Read the model definition and answer for the solid it produces. Units are mm, in the model's axes. A direction names the side the tool comes from. Give positions to 0.01 mm unless a question says otherwise; leave off trailing zeros. Loops run counter-clockwise (first coordinate to the right, second up) from the corner with the lowest first, then second, coordinate; pieces in that order, holes last. Notation, with made-up numbers: (14, -33.5) - (18, -33.5) arc R22 ccw to (18, -4.5) - close; hole circle Ø5 at (15, 44.5). An arc over 180 degrees is marked (long way). Write each question's results on one line, items separated by ' | '. Start each with the question number.
Q1. Determine the mould class of faces 4 (the cylindrical face through (39.563, 38.418, -54.93)), 5 (the flat face through (35.7, 37.6, -30)), 6 (the flat face through (37, 30, -40)), 7 (the flat face through (37, 35, -25)) for opening direction Z: +Z half, -Z half, draft (parallel to the pull), parting line (faces both ways), or undercut.
Q2. The part is cut by section B-B, the plane x = 37.5. Write down the section's boundary in (y, z).
Q3. Find the intervals of material crossed by line 1 (Z direction, x = 37.5, y = 45); line 2 (Y direction, x = 37.5, z = -52.25); line 3 (Y direction, x = 11, z = -52), in increasing order. Write a range as from..to.
Q4. The part is cut by section C-C, the plane y = 40. Write down the section's boundary in (x, z).
Q5. The part is cut by section A-A, the plane z = -37.5. Write down the section's boundary in (x, y).
Q6. For faces 1 (the cylindrical face through (31.5, 24.4, -37.3)), 2 (the flat face through (30, 13, -38)), 3 (the flat face through (17, 5, -80)), determine the directions among +Z, -Z, +X, -X, +Y, -Y from which every point of the face is accessible in a straight line to the end or side of a thin tool.
Q7. The part is cut by section D-D, the plane y = 7. Write down the section's boundary in (x, z), plus the area to 3 significant figures.
Q8. Given pin 1 (10 mm diameter, centred on x = 37.5, y = 26.5, fed in from +Z); pin 2 (1.8 mm diameter, centred on y = 60.5, z = -35.5, fed in from -X); pin 3 (7.5 mm diameter, centred on x = 37.5, y = 39, fed in from -Z), each flat-ended and moving along its own axis, determine where each tip first touches the part or whether it passes through.
```python
from build123d import *

# Parameters (mm, degrees)
SKETCH4_W               = 40
SKETCH4_H               = 80
BOSS_EXTRUDE4_DEPTH     = 5
SKETCH5_W               = 10
SKETCH5_H               = 5
BOSS_EXTRUDE6_DEPTH     = 50
SKETCH7_W               = 10
SKETCH7_H               = 25
SKETCH7_H_2             = 5
BOSS_EXTRUDE7_DEPTH     = 20
SKETCH8_W               = 40
SKETCH8_H               = 5
BOSS_EXTRUDE8_DEPTH     = 20
SKETCH9_W               = 100
SKETCH9_H               = 5
BOSS_EXTRUDE9_DEPTH     = 10
SKETCH10_W              = 5
SKETCH10_H              = 50
BOSS_EXTRUDE10_DEPTH    = 40
BOSS_EXTRUDE11_DEPTH    = 10
SKETCH12_R              = 15
SKETCH12_R_2            = 1.8
CUT_EXTRUDE1_DEPTH      = 5
CUT_EXTRUDE2_DEPTH      = 92.241437954
CUT_EXTRUDE2_DEPTH_BACK = 92.241437954
SKETCH13_R              = 2.25
SKETCH14_R              = 4
SKETCH14_R_2            = 2.25
CUT_EXTRUDE4_DEPTH      = 2
CUT_EXTRUDE5_START      = -2
SKETCH15_R              = 4
SKETCH15_R_2            = 2.25
CUT_EXTRUDE5_DEPTH      = 2
SKETCH17_R              = 5
CUT_EXTRUDE6_DEPTH      = 25
SKETCH19_W              = 50
SKETCH19_H              = 60
SKETCH19_R              = 1.8
SKETCH19_R_2            = 15
SKETCH19_R_3            = 4
BOSS_EXTRUDE13_DEPTH    = 5
SKETCH20_R              = 4
SKETCH20_R_2            = 2.25
BOSS_EXTRUDE14_DEPTH    = 5
SKETCH21_W              = 20
SKETCH21_H              = 20
BOSS_EXTRUDE15_DEPTH    = 5
BOSS_EXTRUDE16_START    = -10
SKETCH22_R              = 4
BOSS_EXTRUDE16_DEPTH    = 10
SKETCH23_R              = 4
BOSS_EXTRUDE17_DEPTH    = 5
CUT_EXTRUDE7_DEPTH      = 106.59356041
CUT_EXTRUDE7_DEPTH_BACK = 106.59356041
SKETCH24_R              = 2.6


with BuildPart() as part:
    # Sketch4 → Boss-Extrude4 (new body)
    with BuildSketch(Plane(origin=(0, 0, 0), x_dir=(1, 0, 0), z_dir=(0, 1, 0))):
        with Locations((20, 40)):
            Rectangle(SKETCH4_W, SKETCH4_H)
    extrude(amount=BOSS_EXTRUDE4_DEPTH)

    # Sketch5 → Boss-Extrude6 (add)
    with BuildSketch(Plane(origin=(0, 5, 0), x_dir=(1, 0, 0), z_dir=(0, 1, 0))):
        with Locations((35, 52.5)):
            Rectangle(SKETCH5_W, SKETCH5_H)
        with Locations((35, 27.5)):
            Rectangle(SKETCH5_W, SKETCH5_H)
    extrude(amount=BOSS_EXTRUDE6_DEPTH)

    # Sketch7 → Boss-Extrude7 (add)
    with BuildSketch(Plane.XY.offset(-50)):
        with Locations((35, 17.5)):
            Rectangle(SKETCH7_W, SKETCH7_H)
        with Locations((35, 52.5)):
            Rectangle(SKETCH7_W, SKETCH7_H_2)
    extrude(amount=BOSS_EXTRUDE7_DEPTH)

    # Sketch8 → Boss-Extrude8 (add)
    with BuildSketch(Plane(origin=(0, 0, -80), x_dir=(-1, 0, 0), z_dir=(0, 0, -1))):
        with Locations((-20, 2.5)):
            Rectangle(SKETCH8_W, SKETCH8_H)
    extrude(amount=BOSS_EXTRUDE8_DEPTH)

    # Sketch9 → Boss-Extrude9 (add)
    with BuildSketch(Plane.ZY):
        with Locations((-50, 2.5)):
            Rectangle(SKETCH9_W, SKETCH9_H)
    extrude(amount=BOSS_EXTRUDE9_DEPTH)

    # Sketch10 → Boss-Extrude10 (add)
    with BuildSketch(Plane.ZY.offset(-30)):
        with Locations((-52.5, 30)):
            Rectangle(SKETCH10_W, SKETCH10_H)
    extrude(amount=BOSS_EXTRUDE10_DEPTH)

    # Sketch11 → Boss-Extrude11 (add)
    with BuildSketch(Plane(origin=(0, 55, 0), x_dir=(1, 0, 0), z_dir=(0, 1, 0))):
        Polygon((40, 55), (-10, 55), (-10, 50), (30, 50), (30, 25), (40, 25), align=None)
    extrude(amount=BOSS_EXTRUDE11_DEPTH)

    # Sketch12 → Cut-Extrude1 (cut)
    with BuildSketch(Plane.XY.offset(-50)):
        with Locations((11, 40)):
            Circle(SKETCH12_R)
        with Locations((-4.499780644, 55.499780644)):
            Circle(SKETCH12_R_2)
        with Locations((26.499780644, 55.499780644)):
            Circle(SKETCH12_R_2)
        with Locations((-4.499780644, 24.500219356)):
            Circle(SKETCH12_R_2)
        with Locations((26.499780644, 24.500219356)):
            Circle(SKETCH12_R_2)
    extrude(amount=-CUT_EXTRUDE1_DEPTH, mode=Mode.SUBTRACT)

    # Sketch13 → Cut-Extrude2 (cut, two sides: drawn at the far end of the back side and taken through both)
    with BuildSketch(Plane.XY.offset(-50).offset(-CUT_EXTRUDE2_DEPTH_BACK)):
        with Locations((35, 40)):
            Circle(SKETCH13_R)
    extrude(amount=CUT_EXTRUDE2_DEPTH + CUT_EXTRUDE2_DEPTH_BACK, mode=Mode.SUBTRACT)

    # Sketch14 → Cut-Extrude4 (cut)
    with BuildSketch(Plane.XY.offset(-25)):
        with Locations((35, 40)):
            Circle(SKETCH14_R)
        with Locations((35, 40)):
            Circle(SKETCH14_R_2, mode=Mode.SUBTRACT)
    extrude(amount=-CUT_EXTRUDE4_DEPTH, mode=Mode.SUBTRACT)

    # Sketch15 → Cut-Extrude5 (cut)
    with BuildSketch(Plane(origin=(0, 0, -55), x_dir=(-1, 0, 0), z_dir=(0, 0, -1)).offset(CUT_EXTRUDE5_START)):
        with Locations(Location((-35, 40, 0), (0, 0, 180))):
            Circle(SKETCH15_R)
        with Locations(Location((-35, 40, 0), (0, 0, 180))):
            Circle(SKETCH15_R_2, mode=Mode.SUBTRACT)
    extrude(amount=CUT_EXTRUDE5_DEPTH, mode=Mode.SUBTRACT)

    # Sketch17 → Cut-Extrude6 (cut)
    with BuildSketch(Plane.XY.offset(-25)):
        with Locations((26.499780644, 55.499780644)):
            Circle(SKETCH17_R)
        with Locations((26.499780644, 24.500219356)):
            Circle(SKETCH17_R)
    extrude(amount=-CUT_EXTRUDE6_DEPTH, mode=Mode.SUBTRACT)

    # Sketch19 → Boss-Extrude13 (add)
    with BuildSketch(Plane(origin=(0, 0, -55), x_dir=(-1, 0, 0), z_dir=(0, 0, -1))):
        with Locations((-15, 35)):
            Rectangle(SKETCH19_W, SKETCH19_H)
        with Locations(Location((4.499780644, 55.499780644, 0), (0, 0, 180))):
            Circle(SKETCH19_R, mode=Mode.SUBTRACT)
        with Locations(Location((4.499780644, 24.500219356, 0), (0, 0, 180))):
            Circle(SKETCH19_R, mode=Mode.SUBTRACT)
        with Locations(Location((-26.499780644, 24.500219356, 0), (0, 0, 180))):
            Circle(SKETCH19_R, mode=Mode.SUBTRACT)
        with Locations(Location((-11, 40, 0), (0, 0, 180))):
            Circle(SKETCH19_R_2, mode=Mode.SUBTRACT)
        with Locations(Location((-35, 40, 0), (0, 0, 180))):
            Circle(SKETCH19_R_3, mode=Mode.SUBTRACT)
        with Locations(Location((-26.499780644, 55.499780644, 0), (0, 0, 180))):
            Circle(SKETCH19_R, mode=Mode.SUBTRACT)
    extrude(amount=BOSS_EXTRUDE13_DEPTH)

    # Sketch20 → Boss-Extrude14 (add)
    with BuildSketch(Plane(origin=(0, 0, -53), x_dir=(-1, 0, 0), z_dir=(0, 0, -1))):
        with Locations(Location((-35, 40, 0), (0, 0, 180))):
            Circle(SKETCH20_R)
        with Locations(Location((-35, 40, 0), (0, 0, 180))):
            Circle(SKETCH20_R_2, mode=Mode.SUBTRACT)
    extrude(amount=BOSS_EXTRUDE14_DEPTH)

    # Sketch21 → Boss-Extrude15 (add)
    with BuildSketch(Plane(origin=(40, 0, 0), x_dir=(0, 0, -1), z_dir=(1, 0, 0))):
        Polygon((100, 5), (60, 5), (60, 65), (25, 65), (25, 5), (0, 5), (0, 0), (100, 0), align=None)
        with Locations((40, 40)):
            Rectangle(SKETCH21_W, SKETCH21_H, mode=Mode.SUBTRACT)
    extrude(amount=BOSS_EXTRUDE15_DEPTH)

    # Sketch22 → Boss-Extrude16 (add)
    with BuildSketch(Plane(origin=(0, 0, -60), x_dir=(-1, 0, 0), z_dir=(0, 0, -1)).offset(BOSS_EXTRUDE16_START)):
        with Locations(Location((-35, 40, 0), (0, 0, 180))):
            Circle(SKETCH22_R)
    extrude(amount=BOSS_EXTRUDE16_DEPTH)

    # Sketch23 → Boss-Extrude17 (add)
    with BuildSketch(Plane.XY.offset(-25)):
        with Locations((35, 40)):
            Circle(SKETCH23_R)
    extrude(amount=-BOSS_EXTRUDE17_DEPTH)

    # Sketch24 → Cut-Extrude7 (cut, two sides: drawn at the far end of the back side and taken through both)
    with BuildSketch(Plane(origin=(0, 0, -30), x_dir=(-1, 0, 0), z_dir=(0, 0, -1)).offset(-CUT_EXTRUDE7_DEPTH_BACK)):
        with Locations((-37.5, 40)):
            Circle(SKETCH24_R)
    extrude(amount=CUT_EXTRUDE7_DEPTH + CUT_EXTRUDE7_DEPTH_BACK, mode=Mode.SUBTRACT)


solid = part.part
```
Check sheet entries:
1) face 4: draft | face 5: undercut | face 6: undercut | face 7: +Z half
2) outline: (0, -100) - (5, -100) - (5, -60) - (37.4, -60) - (37.4, -50) - (30, -50) - (30, -30) - (37.4, -30) - (37.4, -25) - (5, -25) - (5, 0) - (0, 0) - close; (42.6, -60) - (65, -60) - (65, -25) - (42.6, -25) - (42.6, -30) - (50, -30) - (50, -50) - (42.6, -50) - close
3) line 1: z = -60..-50, -30..-25 | line 2: y = 0..37.4, 42.6..65 | line 3: y = 0..25, 55..65
4) outline: (-10, -60) - (-4, -60) - (-4, -50) - (-10, -50) - close; (26, -60) - (34.9, -60) - (34.9, -50) - (26, -50) - close; (30, -30) - (34.9, -30) - (34.9, -25) - (30, -25) - close; (40.1, -60) - (45, -60) - (45, -50) - (40.1, -50) - close; (40.1, -30) - (45, -30) - (45, -25) - (40.1, -25) - close
5) outline: (-10, 0) - (45, 0) - (45, 30) - (30, 30) - (30, 28.07) arc R5 cw to (30, 20.93) - (30, 5) - (-10, 5) - close; (30, 50) - (45, 50) - (45, 65) - (30, 65) - (30, 59.07) arc R5 cw to (30, 51.93) - close
6) face 1: +Z, -X | face 2: +Z, -X, +Y | face 3: -Z, +X, -X, +Y
7) outline: (-10, -60) - (45, -60) - (45, -25) - (30, -25) - (30, -50) - (-10, -50) - close | area: 925 mm^2
8) pin 1: stops at z = -25 | pin 2: stops at x = 30 | pin 3: stops at z = -60
